Design review of the part built by this model. Coordinates are the model's own, in mm. Coordinates: 2 decimals unless noted, no trailing zeros. Write each loop counter-clockwise with the first axis right and the second up, starting at its lowest first coordinate (ties: lowest second). Pieces come first, ordered by that corner, then holes. Notation, with made-up numbers: M -36,-18 L -25,-18 A19 ccw -25,17 Z; hole C 27.5,-8.75 d11. An arc over 180 degrees is marked long. Write item = value, one per line.
```python
from build123d import *

# Parameters (mm, degrees)
SKETCH_11_W         = 20
SKETCH_11_H         = 20
SKETCH_11_W_2       = 18
SKETCH_11_H_2       = 18
F_20X20X1_1_DEPTH   = 360
SKETCH_12_R         = 1.45
CUT_EXTRUDE_1_DEPTH = 34
SKETCH_13_R         = 1.45
CUT_EXTRUDE_2_DEPTH = 361.693775937
CUT_EXTRUDE_3_DEPTH = 361.693775937


with BuildPart() as part:
    # 草图11 → 铝管 20X20X1(1) (new body)
    with BuildSketch(Plane(origin=(0, 0, 0), x_dir=(-1, 0, 0), z_dir=(0, 1, 0))):
        Rectangle(SKETCH_11_W, SKETCH_11_H)
        Rectangle(SKETCH_11_W_2, SKETCH_11_H_2, mode=Mode.SUBTRACT)
    extrude(amount=F_20X20X1_1_DEPTH)

    # 草图12 → 切除-拉伸1 (cut)
    with BuildSketch(Plane(origin=(10, 0, 0), x_dir=(0, 0, -1), z_dir=(1, 0, 0))):
        with Locations((-5, 355)):
            Circle(SKETCH_12_R)
        with Locations((5, 355)):
            Circle(SKETCH_12_R)
        with Locations((-5, 345)):
            Circle(SKETCH_12_R)
        with Locations((5, 345)):
            Circle(SKETCH_12_R)
        with Locations((5, 5)):
            Circle(SKETCH_12_R)
        with Locations((5, 15)):
            Circle(SKETCH_12_R)
        with Locations((5, 25)):
            Circle(SKETCH_12_R)
        with Locations(Location((-5, 5, 0), (0, 0, 180))):
            Circle(SKETCH_12_R)
        with Locations(Location((-5, 15, 0), (0, 0, 180))):
            Circle(SKETCH_12_R)
        with Locations(Location((-5, 25, 0), (0, 0, 180))):
            Circle(SKETCH_12_R)
    extrude(amount=-CUT_EXTRUDE_1_DEPTH, mode=Mode.SUBTRACT)

    # 草图13 → 切除-拉伸2 (cut, through all)
    with BuildSketch(Plane.XY.offset(10)):
        with Locations((-7, 337)):
            Circle(SKETCH_13_R)
        with Locations((7, 337)):
            Circle(SKETCH_13_R)
    extrude(amount=-CUT_EXTRUDE_2_DEPTH, mode=Mode.SUBTRACT)

    # 草图15 → 切除-拉伸3 (cut, through all)
    with BuildSketch(Plane.XY.offset(10)):
        with BuildLine():
            Line((3.5, 33.508109575), (3.5, 7.836953166))
            ThreePointArc((3.5, 7.836953166), (0, 4.336953166), (-3.5, 7.836953166))
            Line((-3.5, 7.836953166), (-3.5, 33.508109575))
            ThreePointArc((-3.5, 33.508109575), (0, 37.008109575), (3.5, 33.508109575))
        make_face()
        with BuildLine():
            Line((-3.5, 46.653630173), (-3.5, 167.118748463))
            ThreePointArc((-3.5, 167.118748463), (0, 170.618748463), (3.5, 167.118748463))
            Line((3.5, 167.118748463), (3.5, 46.653630173))
            ThreePointArc((3.5, 46.653630173), (0, 43.153630173), (-3.5, 46.653630173))
        make_face()
        with BuildLine():
            Line((-3.5, 179.232346303), (-3.5, 315.472332253))
            ThreePointArc((-3.5, 315.472332253), (0, 318.972332253), (3.5, 315.472332253))
            Line((3.5, 315.472332253), (3.5, 179.232346303))
            ThreePointArc((3.5, 179.232346303), (0, 175.732346303), (-3.5, 179.232346303))
        make_face()
        with BuildLine():
            Line((-3.5, 328.562220872), (-3.5, 352.513931961))
            ThreePointArc((-3.5, 352.513931961), (0, 356.013931961), (3.5, 352.513931961))
            Line((3.5, 352.513931961), (3.5, 328.562220872))
            ThreePointArc((3.5, 328.562220872), (0, 325.062220872), (-3.5, 328.562220872))
        make_face()
    extrude(amount=-CUT_EXTRUDE_3_DEPTH, mode=Mode.SUBTRACT)


solid = part.part
```
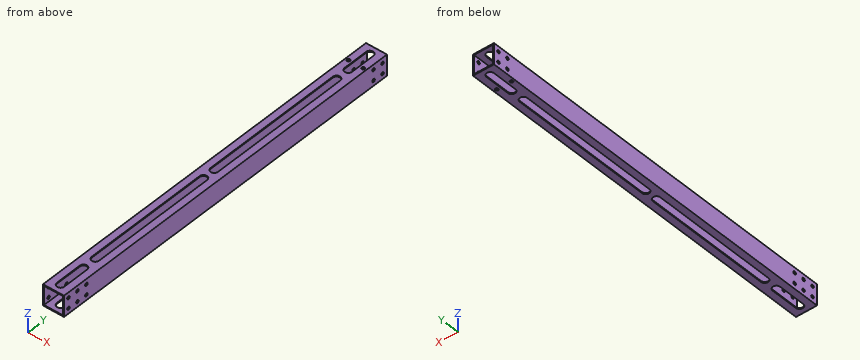
Q1. For P1, Ø2.5, axis at y = 25, z = 5, coming from the -X side, flat-tipped, find the tip position at first contact; note if it passes through.
Check result:
P1 = through
Q2. Consider section C-C, the plane x = 0.5. State how many separate pieces and enclosed holes the cut face has, and give its area (3 significant figures).
Check result:
separate_pieces = 10
enclosed_holes = 0
area = 51.9 mm²
Q3. Wall thickness on line 1 (Z direction, x = -9.25, y = 355); line 2 (Y direction, x = -9.55, z = -5); line 3 (X direction, y = 337, z = -9.6): over which ranges is each line inside the solid? List them lowest first.
Check result:
line_1 = -10 to -6.45, -3.55 to 3.55, 6.45 to 10
line_2 = 0 to 3.55, 6.45 to 13.55, 16.45 to 23.55, 26.45 to 343.55, 346.45 to 353.55, 356.45 to 360
line_3 = -10 to -8.45, -5.55 to -3.5, 3.5 to 5.55, 8.45 to 10
Q4. Consider section A-A, the plane y = 237. State the section outline as (x, z) points.
Check result:
outline = M -10,-10 L -3.5,-10 L -3.5,-9 L -9,-9 L -9,9 L -3.5,9 L -3.5,10 L -10,10 Z; M 3.5,-10 L 10,-10 L 10,10 L 3.5,10 L 3.5,9 L 9,9 L 9,-9 L 3.5,-9 Z
Q5. Consider section B-B, the plane z = 0.5. State the section outline as (x, y) points, and give its area (3 significant figures).
Check result:
outline = M -10,0 L -9,0 L -9,360 L -10,360 Z; M 9,0 L 10,0 L 10,360 L 9,360 Z
area = 720 mm²
